Autodesk Inventor part; units mm, degrees
ref_plane "YZ Plane" through (0, 0, 0) normal (1, 0, 0) x (0, 1, 0)
ref_plane "XZ Plane" through (0, 0, 0) normal (0, 1, 0) x (-1, 0, 0)
ref_plane "XY Plane" through (0, 0, 0) normal (0, 0, 1) x (1, 0, 0)
sketch "Sketch11" plane through (0, 0, 0) normal (0, 1, 0) x (-1, 0, 0)
  circle A0 centre (0, 0) radius 13.75
  line L0 (0, -25.75) -> (7.1, -25.75)
  line L1 (7.1, -25.75) -> (7.1, -19.25)
  line L2 (7.1, -19.25) -> (19, -7.25)
  line L3 (19, -7.25) -> (19, -1.25)
  line L4 (19, -1.25) -> (13.6931, -1.25)
  line L5 (0, -25.75) -> (0, -13.75)
  dimension "d82" = 38
  dimension "d83" = 27.5
  dimension "d84" = 14.2
  dimension "d85" = 6
  dimension "d86" = 12
  dimension "d87" = 6.5
  dimension "d88" = 24.5
extrude "Extrusion7" add sketch "Sketch11" along normal blind 0.8 contours A0 L4 L3 L2 L1 L0 L5
mirror "Mirror5" about plane through (0, 0, -13.75) normal (1, 0, 0) of "Extrusion7"
sketch "Sketch12" plane through (0, 0.8, 0) normal (0, 1, 0) x (1, 0, 0)
  line L0 (-7.1, 25.75) -> (7.1, 25.75)
  line L1 (0, 0) -> (0, 27.3302) construction
  point P0 (-1, 20.25)
  dimension "d91" = 5.5
  dimension "d92" = 1
hole "Hole5" at (-1, 0.8, -20.25) direction (0, -1, 0) diameter 1.2 end through all
pattern_linear "Rectangular Pattern1" count 6 spacing 2 along (1, 0, 0) of "Hole5" first direction both ways yes
sketch "Sketch13" plane through (0, 0, 0) normal (0, -1, 0) x (1, 0, 0)
  circle A0 centre (-17.65, -6.6609) radius 0.75
  circle A1 centre (-7.3109, -17) radius 0.75
  circle A2 centre (7.3109, -17) radius 0.75
  circle A3 centre (17.65, -6.6609) radius 0.75
  point P0 (0, 0)
extrude "Extrusion8" cut sketch "Sketch13" against normal through all
properties part number "Nema 17 PCB" material "MDF Medium Density Fiberboard"
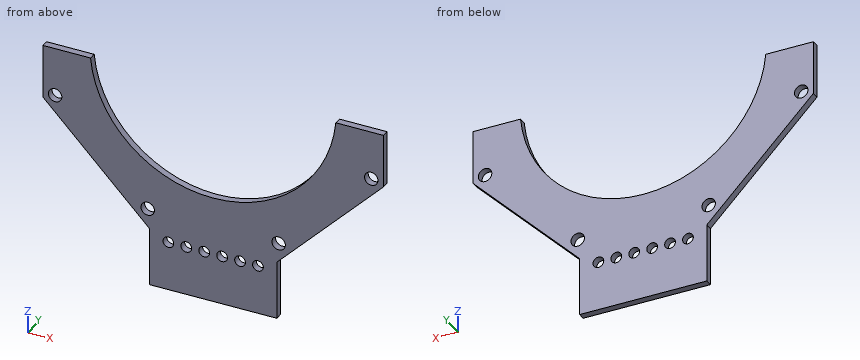
Source: CAD feature listing. Evaluate the final solid. Frame: model axes, mm. Round coordinates to 2 decimals unless told otherwise and drop trailing zeros. Loops run counter-clockwise (first coordinate to the right, second up) from the corner with the lowest first, then second, coordinate; pieces in that order, holes last. Notation, with made-up numbers: (-33.5, 12.25) -> (-13.5, 12.25) arc R9 ccw to (-13.5, 27.25) -> close; hole circle Ø9 at (6, 65). An arc over 180 degrees is marked (long way). Answer as a JSON object with one key per item and string values. Group by question number.
Q1. Section query A-A (x = -1). Output: boundary loops of the cut face in (y, z).
Q2. Section query C-C (y = 0.3). State how many separate pieces and enclosed holes the cut face has, plus the area to 3 significant figures.
Q3. Section query D-D (z = -5). Output: boundary loops of the cut face in (x, y).
Q4. Contact query for a flat-ended pin moving along its axis: P1, Ø0.7, axis at x = 1, z = -20.25, coming from the -Y side. Output: stop coordinate, or through.
Q5. Ray query, line 1 (X direction, y = 0.3, z = -4.25); line 2 (X direction, y = 0.4, z = -21.5); line 3 (X direction, y = 0.4, z = -8.5). Return the intervals inside material, ascending. Write a range as from..to.
Q6. Section query B-B (z = -20.25). Output: boundary loops of the cut face in (x, y).
Completed:
{
 "1": {"outline": "(0, -25.75) -> (0.8, -25.75) -> (0.8, -20.85) -> (0, -20.85) -> close; (0, -19.65) -> (0.8, -19.65) -> (0.8, -13.71) -> (0, -13.71) -> close"},
 "2": {"separate pieces": "1", "enclosed holes": "10", "area": "357 mm²"},
 "3": {"outline": "(-19, 0) -> (-12.81, 0) -> (-12.81, 0.8) -> (-19, 0.8) -> close; (12.81, 0) -> (19, 0) -> (19, 0.8) -> (12.81, 0.8) -> close"},
 "4": {"P1": "through"},
 "5": {"line 1": "-19..-13.08, 13.08..19", "line 2": "-7.1..7.1", "line 3": "-17.76..-10.81, 10.81..17.76"},
 "6": {"outline": "(-7.1, 0) -> (-5.6, 0) -> (-5.6, 0.8) -> (-7.1, 0.8) -> close; (-4.4, 0) -> (-3.6, 0) -> (-3.6, 0.8) -> (-4.4, 0.8) -> close; (-2.4, 0) -> (-1.6, 0) -> (-1.6, 0.8) -> (-2.4, 0.8) -> close; (-0.4, 0) -> (0.4, 0) -> (0.4, 0.8) -> (-0.4, 0.8) -> close; (1.6, 0) -> (2.4, 0) -> (2.4, 0.8) -> (1.6, 0.8) -> close; (3.6, 0) -> (4.4, 0) -> (4.4, 0.8) -> (3.6, 0.8) -> close; (5.6, 0) -> (7.1, 0) -> (7.1, 0.8) -> (5.6, 0.8) -> close"}
}
